from build123d import *

# Parameters (mm, degrees)
F3_R      = 24
F4_DEPTH  = 40
F0_R      = 15
F2_R      = 14.5
F7_DEPTH  = 40.0010001
F9_DEPTH  = 40
F10_W     = 37.1058717763
F10_H     = 24
F11_DEPTH = 85.2906296813
F12_R     = 10
F13_R     = 10


# Not quite as in the source:
# - a pattern or mirror of a feature is missing from the dataset's text; its kind, count and spacing are read off the source's solid


with BuildPart() as f4:
    # F3 (on Top) → F4 (new body)
    with BuildSketch(Plane.XY):
        Circle(F3_R)
    extrude(amount=-F4_DEPTH)

    # F0 (on Top) → F5 section 0
    with BuildSketch(Plane.XY):
        Circle(F0_R)
    # F2 (on offset) → F5 section 1
    with BuildSketch(Plane.XY.offset(-40)):
        Circle(F2_R)
    loft(mode=Mode.SUBTRACT)

    # F6 (on face) → F7 (cut, through all)
    with BuildSketch(Plane.XY):
        with BuildLine():
            Line((-14.2797124187, -4.5923646676), (-14.2797124187, -19.2896296813))
            ThreePointArc((-14.2797124187, -19.2896296813), (0, -24), (14.2797124187, -19.2896296813))
            Line((14.2797124187, -19.2896296813), (14.2797124187, -4.5923646676))
            ThreePointArc((14.2797124187, -4.5923646676), (0, -15), (-14.2797124187, -4.5923646676))
        make_face()
        with BuildLine():
            Line((-14.2797124187, -2.5178985762), (-14.2797124187, -4.5923646676))
            ThreePointArc((-14.2797124187, -4.5923646676), (0, -15), (14.2797124187, -4.5923646676))
            Line((14.2797124187, -4.5923646676), (14.2797124187, -2.5178985762))
            ThreePointArc((14.2797124187, -2.5178985762), (0, -14.5), (-14.2797124187, -2.5178985762))
        make_face()
    extrude(amount=-F7_DEPTH, mode=Mode.SUBTRACT)

    # F8 (on face) → F9 (join)
    with BuildSketch(Plane.XY):
        with BuildLine():
            Line((-14.2797124187, -61.2896296813), (-14.2797124187, -19.2896296813))
            ThreePointArc((-14.2797124187, -19.2896296813), (-21.4326048119, -10.8001597662), (-24, 0))
            Line((-24, 0), (-59.385584195, -61.2896296813))
            Line((-59.385584195, -61.2896296813), (-14.2797124187, -61.2896296813))
        make_face()
        with BuildLine():
            ThreePointArc((24, 0), (21.4326048119, -10.8001597662), (14.2797124187, -19.2896296813))
            Line((14.2797124187, -19.2896296813), (14.2797124187, -61.2896296813))
            Line((14.2797124187, -61.2896296813), (59.385584195, -61.2896296813))
            Line((59.385584195, -61.2896296813), (24, 0))
        make_face()
    extrude(amount=-F9_DEPTH)

    # F10 (on face) → F11 (cut, through all)
    with BuildSketch(Plane.XZ.offset(61.2896296813)):
        with Locations((-40.8326483068, -20)):
            Rectangle(F10_W, F10_H)
    f11 = extrude(amount=-F11_DEPTH, mode=Mode.SUBTRACT)

    # F11_copies: F11 across plane
    add(f11.mirror(Plane(origin=(0, 0, 0), x_dir=(0, 0, 1), z_dir=(1, 0, 0))), mode=Mode.SUBTRACT)

    # F12
    f12_edges = [f4.edges().sort_by_distance(p)[0] for p in [
        (-59.385584, -61.28963, -4),
        (-59.385584, -61.28963, -36),
        (-24, 0, -4),
        (-24, 0, -36),
    ]]
    fillet(f12_edges, radius=F12_R)

    # F13
    f13_edges = [f4.edges().sort_by_distance(p)[0] for p in [
        (59.385584, -61.28963, -4),
        (59.385584, -61.28963, -36),
        (24, 0, -4),
        (24, 0, -36),
    ]]
    fillet(f13_edges, radius=F13_R)


solid = f4.part
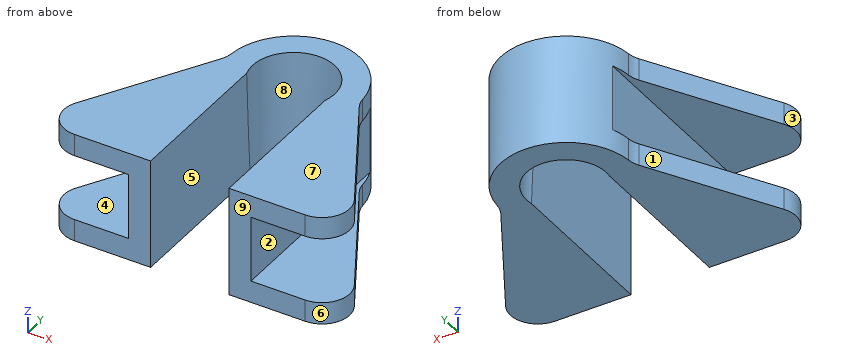
The model under review builds one solid part; all positions refer to its coordinate system, in mm. Face numbers are marked on the shaded views. A direction names the side the tool comes from. Give positions to 0.01 mm unless a question says otherwise; leave off trailing zeros. Write each loop counter-clockwise with the first axis right and the second up, starting at its lowest first coordinate (ties: lowest second). Pieces come first, ordered by that corner, then holes.
1. Add section D-D, the plane y = -18. Write out the cut boundary in (x, z), plus the area to 3 significant figures.
2. Add section A-A, the plane y = -40. Write out the cut boundary in (x, z).
3. Draft analysis for pull direction Y (two halves, no side actions). For the marked faces 6, 7, 8 and 9, state which applies: +Y half, -Y half, draft (parallel to the pull), parting line (faces both ways), or undercut.
4. Tool access review of the marked faces 1, 2, 3, 4 and 5: name each direction out of +Z, -Z, +X, -X, +Y, -Y from which nothing blocks a thin tool from reaching the whole face with its end or side.
5. Wall thickness on L1, parallel to Z at x = 47, y = -52; L2, parallel to X at y = -49.5, z = -30; L3, parallel to X at y = -48, z = -5.5: over which ranges is each line inside the solid? List them lowest first.
6. For P1, Ø1, axis at y = 12, z = -18.5, coming from the -X side; P2, Ø3, axis at y = -52, z = -28, coming from the -X side; P3, Ø10, axis at x = 1.5, z = -32, coming from the -Y side; P4, Ø15, axis at x = -43, y = -26.5, coming from the +Z side, all flat-tipped, find the tip position at first contact; note any pin that passes through.
7. Add section B-B, the plane x = 29. Write out the cut boundary in (y, z).
8. Add section C-C, the plane z = -19.5. Write out the cut boundary in (x, y), plus the area to 3 significant figures.
Worked answers:
1. outline: (-34.39, -40) - (-14.28, -40) - (-14.28, 0) - (-34.39, 0) - (-34.39, -8) - (-22.28, -8) - (-22.28, -32) - (-34.39, -32) - close; (14.28, -40) - (34.39, -40) - (34.39, -32) - (22.28, -32) - (22.28, -8) - (34.39, -8) - (34.39, 0) - (14.28, 0) - close
1. area: 1,030 mm2
2. outline: (-47.09, -40) - (-14.28, -40) - (-14.28, 0) - (-47.09, 0) - (-47.09, -8) - (-22.28, -8) - (-22.28, -32) - (-47.09, -32) - close; (14.28, -40) - (47.09, -40) - (47.09, -32) - (22.28, -32) - (22.28, -8) - (47.09, -8) - (47.09, 0) - (14.28, 0) - close
3. face 6: parting line
3. face 7: draft
3. face 8: undercut
3. face 9: -Y half
4. face 1: +Z, -Z, -X, +Y
4. face 2: +X, +Y, -Y
4. face 3: +Z, -Z, -X
4. face 4: -X, +Y, -Y
4. face 5: +Z, -Z, -Y
5. L1: z = -40 to -32, -8 to 0
5. L2: x = -22.28 to -14.28, 14.28 to 22.28
5. L3: x = -51.51 to -14.28, 14.28 to 51.51
6. P1: stops at x = -21.07
6. P2: stops at x = -22.28
6. P3: stops at y = 13.07
6. P4: stops at z = 0
7. outline: (-61.29, -40) - (-8.66, -40) - (-8.66, -32) - (-61.29, -32) - close; (-61.29, -8) - (-8.66, -8) - (-8.66, 0) - (-61.29, 0) - close
8. outline: (-22.28, -61.29) - (-14.28, -61.29) - (-14.28, -3.72) arc R14.76 cw (long way) to (14.28, -3.72) - (14.28, -61.29) - (22.28, -61.29) - (22.28, 8.92) arc R24 ccw to (-22.28, 8.92) - close
8. area: 1,520 mm2
